The listing builds one solid part. Answer for the finished solid, in the listing's coordinates (mm). Face numbers are marked on the shaded views. A direction names the side the tool comes from. Round coordinates to 2 decimals unless told otherwise and drop trailing zeros. Order: outer loops, then holes, each group sorted by start corner. A loop starts at its lowest first (then second) coordinate and runs counter-clockwise, first axis right, second up. Notation, with made-up numbers: (31, 72.5) - (90, 72.5) arc R22 cw to (90, 82.5) - close; hole circle Ø4 at (7.5, -19.75). An arc over 180 degrees is marked (long way). Use CSV: the item, a comma, the result in double quotes. Start each with the question number.
Item 1: Determine the mould class of the marked faces 3, 4, 5 and 6 for opening direction Y: +Y half, -Y half, draft (parallel to the pull), parting line (faces both ways), or undercut.
Item 2: Find section B-B, the plane y = 0. Give the vertices of the cut face in (x, z), plus the area to 3 significant figures.
Item 3: Find section A-A, the plane x = -20.72. Give the vertices of the cut face in (y, z) (3 decimals), plus the area to 4 significant figures.
Item 4: Flat-ended cylindrical pins translate along their axes: P1, Ø5.5, axis at y = 0.5, z = 2, coming from the +X side; P2, Ø13.5, axis at x = 0.5, z = -17, coming from the -Y side; P3, Ø1.5, axis at x = -20.5, y = 5.5, coming from the -Z side. Find the tip coordinate at first contact, or state that the pin passes through.
Item 5: Find section D-D, the plane y = 7.62. Give the vertices of the cut face in (x, z) (3 decimals).
Item 6: For the marked faces 1 and 2, determine the directions among +Z, -Z, +X, -X, +Y, -Y from which every point of the face is accessible in a straight line to the end or side of a thin tool.
Item 7: Find section C-C, the plane z = -12.5. Give the vertices of the cut face in (x, y).
Item 8: Straight lines are drawn through the part: line 1 along Y through (x, z) = (-18, 3); line 2 along Y through (x, z) = (20.5, -2.5); line 3 along X through (y, z) = (6.55, -26). For each, find the intervals that lie inside material, in ascending order. Write a range as [from, to].
```python
from build123d import *

# Parameters (mm, degrees)
SKETCH_1_W          = 44
SKETCH_1_H          = 18
SKETCH_1_R          = 5
EXTRUDE_1_DEPTH     = 4
SKETCH_2_W          = 10
SKETCH_2_H          = 9
CUT_EXTRUDE_1_DEPTH = 25.103941586
SKETCH_3_R          = 0.875
EXTRUDE_2_DEPTH     = 5.5
SKETCH_4_W          = 41
SKETCH_4_H          = 4
EXTRUDE_3_DEPTH     = 30
SKETCH_5_R          = 7.35
EXTRUDE_4_DEPTH     = 3
CUT_EXTRUDE_2_DEPTH = 40.749213829
EXTRUDE_6_DEPTH     = 4
SKETCH_8_R          = 1.75
CUT_EXTRUDE_3_DEPTH = 43.087666423
CHAMFER_1_SIZE      = 3
SKETCH_9_R          = 2.5
CUT_EXTRUDE_5_DEPTH = 45.445153447
CHAMFER_2_SIZE      = 4


with BuildPart() as part:
    # Эскиз1 → Бобышка-Вытянуть1 (new body)
    with BuildSketch(Plane.XY):
        Rectangle(SKETCH_1_W, SKETCH_1_H)
        Circle(SKETCH_1_R, mode=Mode.SUBTRACT)
    extrude(amount=EXTRUDE_1_DEPTH)

    # Эскиз2 → Вырез-Вытянуть1 (cut, through all)
    with BuildSketch(Plane.XY.offset(4)):
        with Locations((-17, 0)):
            Rectangle(SKETCH_2_W, SKETCH_2_H)
    extrude(amount=-CUT_EXTRUDE_1_DEPTH, mode=Mode.SUBTRACT)

    # Эскиз3 → Бобышка-Вытянуть2 (add)
    with BuildSketch(Plane.XY.offset(4)):
        with Locations((-20.72, 7.62)):
            Circle(SKETCH_3_R)
        with Locations((-20.72, -7.62)):
            Circle(SKETCH_3_R)
        with Locations((19.92, -7.62)):
            Circle(SKETCH_3_R)
        with Locations((19.92, 7.62)):
            Circle(SKETCH_3_R)
    extrude(amount=EXTRUDE_2_DEPTH)

    # Эскиз4 → Бобышка-Вытянуть3 (add)
    with BuildSketch(Plane(origin=(0, 0, 0), x_dir=(-1, 0, 0), z_dir=(0, 0, -1))):
        with Locations((-1.5, 7)):
            Rectangle(SKETCH_4_W, SKETCH_4_H)
    extrude(amount=EXTRUDE_3_DEPTH)

    # Эскиз5 → Бобышка-Вытянуть4 (add)
    with BuildSketch(Plane(origin=(0, 9, 0), x_dir=(1, 0, 0), z_dir=(0, 1, 0))):
        with Locations(Location((-5.61, 15.5, 0), (0, 0, 90))):
            Circle(SKETCH_5_R)
    extrude(amount=EXTRUDE_4_DEPTH)

    # Эскиз6 → Вырез-Вытянуть2 (cut, through all)
    with BuildSketch(Plane.XZ.offset(-5)):
        Polygon((22, -3.01), (6.48, -30), (22, -30), align=None)
    extrude(amount=-CUT_EXTRUDE_2_DEPTH, mode=Mode.SUBTRACT)

    # Эскиз7 → Бобышка-Вытянуть6 (add)
    with BuildSketch(Plane.XZ.offset(-5)):
        Polygon((25.987913824, -9.945167145), (22, -3.01), (16.087917757, -13.291385293), (20.07583158, -20.226552439), align=None)
    extrude(amount=-EXTRUDE_6_DEPTH)

    # Эскиз8 → Вырез-Вытянуть3 (cut, through all)
    with BuildSketch(Plane.XZ.offset(-5)):
        with Locations(Location((21.03791579, -11.618276219, 0), (0, 0, 270))):
            Circle(SKETCH_8_R)
        with Locations(Location((-12, -26, 0), (0, 0, 270))):
            Circle(SKETCH_8_R)
        with Locations(Location((1.48, -26, 0), (0, 0, 270))):
            Circle(SKETCH_8_R)
        with Locations(Location((6, -9, 0), (0, 0, 270))):
            Circle(SKETCH_8_R)
    extrude(amount=-CUT_EXTRUDE_3_DEPTH, mode=Mode.SUBTRACT)

    # Фаска1
    # the kernel refuses this chamfer: 3 mm, written as the material it adds along each edge
    with BuildSketch(Plane(origin=(2.6e-08, 5, 0), x_dir=(0, -0.9996219169112968, 0.027495876610586372), z_dir=(-1, 0, 0))) as chamfer_1_piece_1_section:
        Polygon((CHAMFER_1_SIZE * 0.999621916911, -CHAMFER_1_SIZE * 0.0274958766106), (-CHAMFER_1_SIZE * 0.0274958766106, -CHAMFER_1_SIZE * 0.999621916911), (0, 0), align=None)
    chamfer_1_piece_1 = extrude(amount=26.71504899, mode=Mode.PRIVATE)
    chamfer_1_piece_1 = split(chamfer_1_piece_1, bisect_by=Plane(origin=(-12, 3.70825936, -0.85412968), z_dir=(1, 0, 0)), keep=Keep.TOP, mode=Mode.PRIVATE)
    chamfer_1_piece_1 = chamfer_1_piece_1 - Plane(origin=(0, 0, -0.85412968), x_dir=(1, 0, 0), z_dir=(0, 0, -1)) * Cylinder(5, 66, mode=Mode.PRIVATE)
    add(chamfer_1_piece_1)
    with BuildSketch(Plane(origin=(2.6e-08, 5, 0), x_dir=(0, -0.9996219169112968, 0.027495876610586372), z_dir=(-1, 0, 0))) as chamfer_1_piece_2_section:
        Polygon((CHAMFER_1_SIZE * 0.999621916911, -CHAMFER_1_SIZE * 0.0274958766106), (-CHAMFER_1_SIZE * 0.0274958766106, -CHAMFER_1_SIZE * 0.999621916911), (0, 0), align=None)
    chamfer_1_piece_2 = extrude(amount=19.000000026, mode=Mode.PRIVATE)
    chamfer_1_piece_2 = split(chamfer_1_piece_2, bisect_by=Plane(origin=(-15.5, 4.5, -1.378787879), z_dir=(0, 1, 0)), keep=Keep.TOP, mode=Mode.PRIVATE)
    chamfer_1_piece_2 = split(chamfer_1_piece_2, bisect_by=Plane(origin=(-12, 4.757575758, -1.378787879), z_dir=(-1, 0, 0)), keep=Keep.TOP, mode=Mode.PRIVATE)
    add(chamfer_1_piece_2)
    with BuildSketch(Plane(origin=(22, 5, 0), x_dir=(0, -0.9996219169112968, 0.027495876610586372), z_dir=(-1, 0, 0))) as chamfer_1_piece_3_section:
        Polygon((CHAMFER_1_SIZE * 0.999621916911, -CHAMFER_1_SIZE * 0.0274958766106), (-CHAMFER_1_SIZE * 0.0274958766106, -CHAMFER_1_SIZE * 0.999621916911), (0, 0), align=None)
    chamfer_1_piece_3 = extrude(amount=21.999999974, mode=Mode.PRIVATE)
    chamfer_1_piece_3 = chamfer_1_piece_3 - Plane(origin=(0, 0, -1.018193592), x_dir=(1, 0, 0), z_dir=(0, 0, -1)) * Cylinder(5, 56, mode=Mode.PRIVATE)
    add(chamfer_1_piece_3)

    # Эскиз9 → Вырез-Вытянуть5 (cut, through all)
    with BuildSketch(Plane.XY.offset(4)):
        with Locations((13, 0)):
            Circle(SKETCH_9_R)
    extrude(amount=-CUT_EXTRUDE_5_DEPTH, mode=Mode.SUBTRACT)

    # Фаска2
    chamfer_2_edges = [part.edges().sort_by_distance(p)[0] for p in [
        (-19, 7, -30),
    ]]
    chamfer(chamfer_2_edges, length=CHAMFER_2_SIZE)


solid = part.part
```
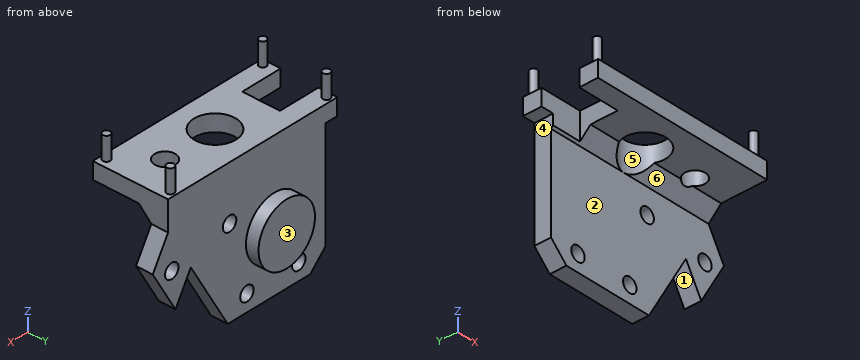
Worked out:
1,face 3,"+Y half"
1,face 4,"draft"
1,face 5,"undercut"
1,face 6,"-Y half"
2,outline,"(-12, 0) - (-5, 0) - (-5, 4) - (-12, 4) - close; (5, 0) - (10.5, 0) - (10.5, 4) - (5, 4) - close; (15.5, 0) - (22, 0) - (22, 4) - (15.5, 4) - close"
2,area,"76.0 mm²"
3,outline,"(-9, 0) - (-4.5, 0) - (-4.5, 4) - (-6.745, 4) - (-6.745, 9.5) - (-8.495, 9.5) - (-8.495, 4) - (-9, 4) - close; (4.5, 0) - (9, 0) - (9, 4) - (8.495, 4) - (8.495, 9.5) - (6.745, 9.5) - (6.745, 4) - (4.5, 4) - close"
3,area,"55.25 mm²"
4,P1,"stops at x = 22"
4,P2,"stops at y = 5"
4,P3,"stops at z = 0"
5,outline,"(-22, 0) - (-19, 0) - (-19, -26) - (-15, -30) - (6.48, -30) - (16.088, -13.291) - (20.076, -20.227) - (25.988, -9.945) - (22, -3.01) - (22, 4) - (20.795, 4) - (20.795, 9.5) - (19.045, 9.5) - (19.045, 4) - (-19.845, 4) - (-19.845, 9.5) - (-21.595, 9.5) - (-21.595, 4) - (-22, 4) - close; hole circle Ø3.5 at (-12, -26); hole circle Ø3.5 at (1.48, -26); hole circle Ø3.5 at (6, -9); hole circle Ø3.5 at (21.038, -11.618)"
6,face 1,"-Z, +Y, -Y"
6,face 2,"-Z, +X, -X, -Y"
7,outline,"(-19, 5) - (19.53, 5) - (19.53, 9) - (1.1, 9) - (1.1, 12) - (-12.32, 12) - (-12.32, 9) - (-19, 9) - close; (22.55, 5) - (24.52, 5) - (24.52, 9) - (22.55, 9) - close"
8,line 1,"y = [-9, -4.5], [4.5, 9]"
8,line 2,"y = [4.5, 9]"
8,line 3,"x = [-19, -13.75], [-10.25, -0.27], [3.23, 8.78]"
